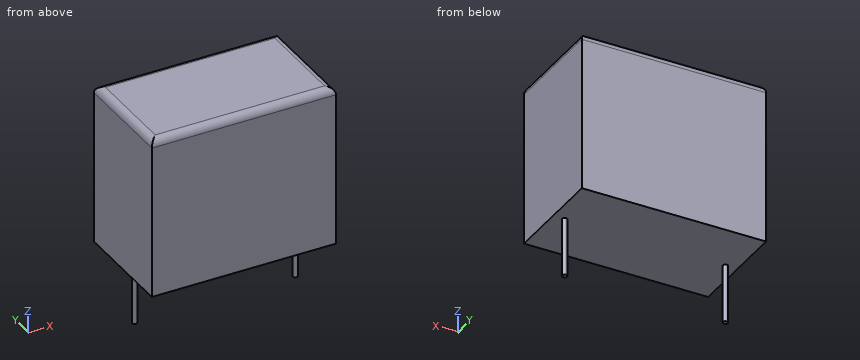
```python
from build123d import *

# Parameters (mm, degrees)
F0_W     = 31.5
F0_H     = 18
F0_R     = 0.4
F1_DEPTH = 27.5
F2_R     = 0.4
F3_DEPTH = 10
F4_R     = 1.27


with BuildPart() as f1:
    # F0 (on Top) → F1 (new body)
    with BuildSketch(Plane.XY):
        Rectangle(F0_W, F0_H)
        with Locations((-13.75, 0)):
            Circle(F0_R, mode=Mode.SUBTRACT)
        with Locations((13.75, 0)):
            Circle(F0_R, mode=Mode.SUBTRACT)
        with Locations((13.75, 0)):
            Circle(F0_R)
        with Locations((-13.75, 0)):
            Circle(F0_R)
    extrude(amount=F1_DEPTH)

    # F2 (on face) → F3 (join)
    with BuildSketch(Plane(origin=(0, 0, 0), x_dir=(1, 0, 0), z_dir=(0, 0, -1))):
        with Locations((13.75, 0)):
            Circle(F2_R)
        with Locations((-13.75, 0)):
            Circle(F2_R)
    extrude(amount=F3_DEPTH)

    # F4
    f4_edges = [f1.edges().sort_by_distance(p)[0] for p in [
        (-15.75, 0, 27.5),
        (0, -9, 27.5),
        (15.75, 0, 27.5),
        (0, 9, 27.5),
    ]]
    fillet(f4_edges, radius=F4_R)


solid = f1.part
```
For this review, take the finished solid that the model builds, in its own axes (mm). Coordinates: 2 decimals unless noted, no trailing zeros. Write each loop counter-clockwise with the first axis right and the second up, starting at its lowest first coordinate (ties: lowest second). Pieces come first, ordered by that corner, then holes. Notation, with made-up numbers: (-23, 25) - (4, 25) arc R31 ccw to (4, 53) - close; hole circle Ø4 at (-29, 54.5). An arc over 180 degrees is marked (long way). Put each result on its own line as item: value.
1. Add section B-B, the plane y = -3.75. Give the boundary of the cut face in (x, z), then the cut area to 3 significant figures.
Values found:
outline: (-15.75, 0) - (15.75, 0) - (15.75, 26.23) arc R1.27 ccw to (14.48, 27.5) - (-14.48, 27.5) arc R1.27 ccw to (-15.75, 26.23) - close
area: 866 mm²
2. Add section A-A, the plane x = 7. Give the boundary of the cut face in (y, z).
Values found:
outline: (-9, 0) - (9, 0) - (9, 26.23) arc R1.27 ccw to (7.73, 27.5) - (-7.73, 27.5) arc R1.27 ccw to (-9, 26.23) - close
3. Wall thickness on probe 1 along Z at (x, y) = (1, -0.5); probe 2 along X at (y, z) = (-0.25, -6.5); probe 3 along Y at (x, z) = (-13.5, -3.5): over which ranges is each line inside the solid? List them lowest first.
Values found:
probe 1: 0 to 27.5
probe 2: -14.06 to -13.44, 13.44 to 14.06
probe 3: -0.31 to 0.31
4. For pin 1 (10 mm diameter, centred on x = 5.5, y = 1, fed in from -Z), flat-tipped, find the tip position at first contact; note if it passes through.
Values found:
pin 1: z = 0
